Geometry: final body of the model. Coordinates: model frame, mm. Give positions to 0.01 mm unless a question says otherwise; leave off trailing zeros. Loops run counter-clockwise (first coordinate to the right, second up) from the corner with the lowest first, then second, coordinate; pieces in that order, holes last. Notation, with made-up numbers: (63.5, 55) - (71.5, 55) arc R19 cw to (71.5, 89) - close; hole circle Ø2 at (59.5, 62.25). An arc over 180 degrees is marked (long way). Use one line per item in the form item = value.
```python
from build123d import *

# Parameters (mm, degrees)
SKETCH1_R          = 3.3274
EXTRUDE3_DEPTH     = 1.524
SKETCH4_W          = 12.7
SKETCH4_H          = 1.7526
CHAMFER1_SIZE      = 0.5953125
SKETCH26_R         = 0.8763
EXTRUDE8_DEPTH     = 1.524
CUT_EXTRUDE3_REACH = 15.544
CIRPATTERN1_COUNT  = 4
DRAFT2_ANGLE       = 5


# Read off the part's stored shape, not the designer's step: Extrude10, Draft1
with BuildPart() as part:
    # Sketch1 → Extrude3 (new body)
    with BuildSketch(Plane.XY):
        with Locations(Location((0, 0, 0), (0, 0, 180))):
            Circle(SKETCH1_R)
    extrude(amount=EXTRUDE3_DEPTH)

    # Sketch11 → Cut-Revolve3 (revolve, cut)
    with BuildSketch(Plane(origin=(0, 0, 0), x_dir=(0, 0, -1), z_dir=(1, 0, 0)), mode=Mode.PRIVATE) as cut_revolve3_sk:
        Polygon((0, 1.511167525), (-1.524, 3.3274), (0, 3.3274), align=None)
    revolve(cut_revolve3_sk.sketch.rotate(Axis((0, 0, -0.441444004), (0, 0, 1)), 90), axis=Axis((0, 0, -0.441444004), (0, 0, 1)), mode=Mode.SUBTRACT)

    # Extrude10 outline → Extrude10 (revolve)
    with BuildSketch(Plane.XZ):
        Polygon((1.7526, 0), (1.7526, 0.202585901), (1.511167525, 0.202585901), (1.511167525, 0), (0, 0), (0, -1.7526), align=None)
    revolve(axis=Axis((0, 0, 0), (0, 0, 1)))



with BuildPart() as body_2:
    # Sketch4 → Revolve1 (revolve)
    with BuildSketch(Plane(origin=(0, 0, 0), x_dir=(0, 0, -1), z_dir=(1, 0, 0)), mode=Mode.PRIVATE) as revolve1_sk:
        with Locations((4.826, 0.8763)):
            Rectangle(SKETCH4_W, SKETCH4_H)
    revolve(revolve1_sk.sketch.rotate(Axis((0, 0, 1.524), (0, 0, -1)), 180), axis=Axis((0, 0, 1.524), (0, 0, -1)))

    # Chamfer1
    chamfer1_edges = [body_2.edges().sort_by_distance(p)[0] for p in [
        (0, 1.7526, -11.176),
    ]]
    chamfer(chamfer1_edges, length=CHAMFER1_SIZE)


with BuildPart() as part_1:
    add(part.part)

    add(body_2.part)  # Extrude8 merges body 2
    # Sketch26 → Extrude8 (add)
    with BuildSketch(Plane.XY.offset(1.524)):
        Circle(SKETCH26_R)
    extrude(amount=-EXTRUDE8_DEPTH)

    # Cut-Extrude3: up to this cone (the profile starts inside it)
    cut_extrude3_end = Plane(origin=(0, 0, 1.524), z_dir=(0, 0, 1)).offset(-2.068083744) * Cone(1.192e-06, 24.522394484, 20.576731167, align=(Align.CENTER, Align.CENTER, Align.MIN), mode=Mode.PRIVATE)
    # Sketch12 → Cut-Extrude3 (cut, up to the surface)
    with BuildSketch(Plane.XY.offset(1.524), mode=Mode.PRIVATE) as cut_extrude3_sk1:
        with BuildLine():
            Line((2.173448579, 0.443653333), (1.308550956, 0.443653333))
            Line((1.308550956, 0.443653333), (0.696975982, 0.696975982))
            Line((0.696975982, 0.696975982), (0.443653333, 1.308550956))
            Line((0.443653333, 1.308550956), (0.443653333, 2.173448579))
            ThreePointArc((0.443653333, 2.173448579), (0.22295568, 2.207033704), (0, 2.218266667))
            Line((0, 2.218266667), (0, 0))
            Line((0, 0), (2.218266667, 0))
            ThreePointArc((2.218266667, 0), (2.207033704, 0.22295568), (2.173448579, 0.443653333))
        make_face()
    cut_extrude3_tool1 = extrude(cut_extrude3_sk1.sketch, amount=-CUT_EXTRUDE3_REACH, mode=Mode.PRIVATE) & cut_extrude3_end
    cut_extrude3 = cut_extrude3_tool1.solids().sort_by_distance((1.741, 0.412282, 1.524))[0]
    add(cut_extrude3, mode=Mode.SUBTRACT)

    # CirPattern1: Cut-Extrude3 ×4 about axis
    cirpattern1_axis = Axis((0, 0, 0), (0, 0, 1))
    for i in range(1, CIRPATTERN1_COUNT):
        add(cut_extrude3.rotate(cirpattern1_axis, i * 360 / CIRPATTERN1_COUNT), mode=Mode.SUBTRACT)

    # Draft1 outline → Draft1 (revolve)
    with BuildSketch(Plane.XZ):
        Polygon((2.218266667, 1.524), (2.146804001, 1.257297702), (2.218266667, 1.257297702), align=None)
    revolve(axis=Axis((0, 0, 0), (0, 0, 1)))

    # Draft2
    draft2_faces = [part_1.faces().sort_by_distance(p)[0] for p in [
        (0.443653333, 1.642629798, 1.204938596),
        (0.576807254, 0.987088954, 0.973802508),
        (0.987088954, 0.576807254, 0.973802508),
        (1.642629798, 0.443653333, 1.204938596),
        (1.642629798, -0.443653333, 1.204938596),
        (0.987088954, -0.576807254, 0.973802508),
        (0.576807254, -0.987088954, 0.973802508),
        (0.443653333, -1.642629798, 1.204938596),
        (-0.443653333, -1.642629798, 1.204938596),
        (-0.576807254, -0.987088954, 0.973802508),
        (-0.987088954, -0.576807254, 0.973802508),
        (-1.642629798, -0.443653333, 1.204938596),
        (-1.642629798, 0.443653333, 1.204938596),
        (-0.987088954, 0.576807254, 0.973802508),
        (-0.576807254, 0.987088954, 0.973802508),
        (-0.443653333, 1.642629798, 1.204938596),
    ]]
    draft(draft2_faces, Plane(origin=(0, 1.7526, 1.524), x_dir=(0, 1, 0), z_dir=(0, 0, 1)), DRAFT2_ANGLE)


solid = part_1.part
```
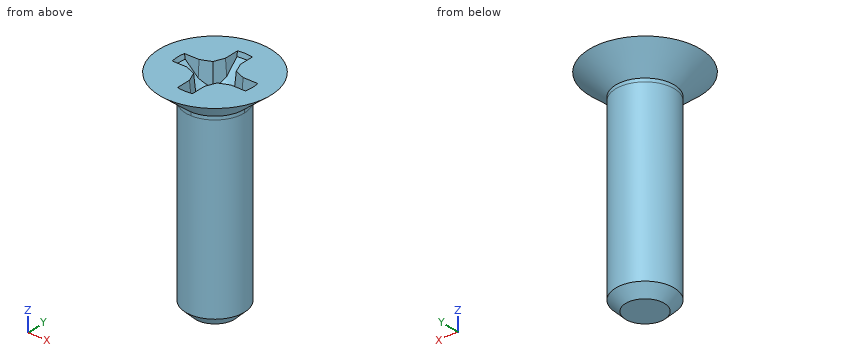
(1) Cut plane A-A (z = -10.25). Return the cut outline in (x, y), plus the area to 3 significant figures.
Solution:
outline = circle Ø3.51 at (0, 0)
area = 9.65 mm2
(2) Material intervals for L1, parallel to Z at x = 0.5, y = 2.75; L2, parallel to Z at x = 2.25, y = -1; L3, parallel to Y at x = -1.25, z = 0.25, sorted ascending. Write a range as from..to.
Solution:
L1 = 1.08..1.52
L2 = 0.8..1.52
L3 = -1.31..1.31
(3) Pin query (flat end, axial travel): P1, Ø3, axis at y = 1, z = -4, coming from the +X side. Return the tip coordinate at first contact, or that it passes through.
Solution:
P1 = 1.75
